from build123d import *

# Parameters (mm, degrees)
SKETCH_1_R          = 8.3
EXTRUDE_1_DEPTH     = 4.5
SKETCH_2_R          = 6.1
CUT_EXTRUDE_1_DEPTH = 1.4
SKETCH_3_R          = 7
EXTRUDE_4_DEPTH     = 13
SKETCH_9_R          = 2.5
CUT_EXTRUDE_7_DEPTH = 22.072019362
CUT_EXTRUDE_START   = -13
CUT_EXTRUDE_8_DEPTH = 13
SKETCH_12_R         = 3.15
CUT_EXTRUDE_9_DEPTH = 7


with BuildPart() as part:
    # Эскиз1 → Бобышка-Вытянуть1 (new body)
    with BuildSketch(Plane(origin=(0, 0, 0), x_dir=(0, 0, -1), z_dir=(1, 0, 0))):
        Circle(SKETCH_1_R)
    extrude(amount=EXTRUDE_1_DEPTH)

    # Эскиз2 → Вырез-Вытянуть1 (cut)
    with BuildSketch(Plane.ZY):
        with Locations((-0.21618585, 0)):
            Circle(SKETCH_2_R)
    extrude(amount=-CUT_EXTRUDE_1_DEPTH, mode=Mode.SUBTRACT)

    # Эскиз3 → Бобышка-Вытянуть4 (add)
    with BuildSketch(Plane(origin=(4.5, 0, 0), x_dir=(0, 0, -1), z_dir=(1, 0, 0))):
        with Locations(Location((0, 0, 0), (0, 0, 180))):
            Circle(SKETCH_3_R)
    extrude(amount=EXTRUDE_4_DEPTH)

    # Эскиз9 → Вырез-Вытянуть7 (cut, through all)
    with BuildSketch(Plane(origin=(17.5, 0, 0), x_dir=(0, 0, -1), z_dir=(1, 0, 0))):
        Circle(SKETCH_9_R)
    extrude(amount=-CUT_EXTRUDE_7_DEPTH, mode=Mode.SUBTRACT)

    # Эскиз10 → Вырез-Вытянуть8 (cut)
    with BuildSketch(Plane(origin=(17.5, 0, 0), x_dir=(0, 0, -1), z_dir=(1, 0, 0)).offset(CUT_EXTRUDE_START)):
        with BuildLine():
            Line((-4, -5.744562647), (4, -5.744562647))
            ThreePointArc((4, -5.744562647), (0, -7), (-4, -5.744562647))
        make_face()
    extrude(amount=CUT_EXTRUDE_8_DEPTH, mode=Mode.SUBTRACT)

    # Эскиз12 → Вырез-Вытянуть9 (cut)
    with BuildSketch(Plane.ZY):
        Circle(SKETCH_12_R)
    extrude(amount=-CUT_EXTRUDE_9_DEPTH, mode=Mode.SUBTRACT)


solid = part.part
Source: CAD feature listing. Evaluate the final solid. Frame: model axes, mm. A direction names the side the tool comes from. Coordinates: 2 decimals unless noted, no trailing zeros. Order: outer loops, then holes, each group sorted by start corner. A loop starts at its lowest first (then second) coordinate and runs counter-clockwise, first axis right, second up.
Item 1: First-contact query: P1, Ø2, axis at x = 12.5, y = 5, coming from the +Z side; P2, Ø1, axis at x = 15.5, z = 3, coming from the +Y side; P3, Ø1, axis at x = 8.5, z = -1, coming from the +Y side; P4, Ø4.5, axis at y = 0, z = 0, coming from the -X side. Flat tips, straight axial feed; report the tip coordinate or a pass-through.
Output values:
P1: stops at z = 5.74
P2: stops at y = 6.54
P3: stops at y = 6.98
P4: passes through
Item 2: Cut plane D-D (z = 0). Return loops of the section in (x, y).
Output values:
outline: (0, -8.3) - (4.5, -8.3) - (4.5, -5.74) - (17.5, -5.74) - (17.5, -2.5) - (7, -2.5) - (7, -3.15) - (1.4, -3.15) - (1.4, -6.1) - (0, -6.1) - close; (0, 6.1) - (1.4, 6.1) - (1.4, 3.15) - (7, 3.15) - (7, 2.5) - (17.5, 2.5) - (17.5, 7) - (4.5, 7) - (4.5, 8.3) - (0, 8.3) - close
Item 3: Pull-direction query (Y, two-part tool) for faces 4 (the face through (4.5, -6, 0)), 5 (the face through (11, -5.745, 0)), 6 (the face through (7, 2, -2)); classes: pulls with the +Y half, pulls with the -Y half, needs draft (parallel to the pull), parting line crosses it, or undercut.
Output values:
face 4: needs draft
face 5: pulls with the -Y half
face 6: undercut
Item 4: Material intervals for line 1 (Y direction, x = 5, z = 0); line 2 (Y direction, x = 2.9, z = 0); line 3 (X direction, y = 5.25, z = -1.75), sorted ascending.
Output values:
line 1: y = -5.74 to -3.15, 3.15 to 7
line 2: y = -8.3 to -3.15, 3.15 to 8.3
line 3: x = 1.4 to 17.5
Item 5: Set-up query: faces 1 (the face through (12.32, -2.44, 0.54)), 2 (the face through (1.4, 1.4, -3)), 3 (the face through (11, 7, 0)). Return all of +Z, -Z, +X, -X, +Y, -Y with unobstructed straight access to the full face (end or side cutting, diameter ignored); none if empty.
Output values:
face 1: +X, -X
face 2: -X
face 3: +X
Item 6: Cut plane A-A (y = 0). Return loops of the section in (x, z), plus the area to 3 significant figures.
Output values:
outline: (0, -8.3) - (4.5, -8.3) - (4.5, -7) - (17.5, -7) - (17.5, -2.5) - (7, -2.5) - (7, -3.15) - (1.4, -3.15) - (1.4, -6.32) - (0, -6.32) - close; (0, 5.88) - (1.4, 5.88) - (1.4, 3.15) - (7, 3.15) - (7, 2.5) - (17.5, 2.5) - (17.5, 7) - (4.5, 7) - (4.5, 8.3) - (0, 8.3) - close
area: 152 mm2
Item 7: Cut plane B-B (z = 5.25). Return loops of the section in (x, y).
Output values:
outline: (0, -6.43) - (4.5, -6.43) - (4.5, -4.63) - (17.5, -4.63) - (17.5, 4.63) - (4.5, 4.63) - (4.5, 6.43) - (0, 6.43) - (0, 2.71) - (1.4, 2.71) - (1.4, -2.71) - (0, -2.71) - close
Item 8: Cut plane C-C (x = 8.25). Return loops of the section in (y, z).
Output values:
outline: (-5.74, -4) arc R7 ccw (long way) to (-5.74, 4) - close; hole circle Ø5 at (0, 0)
